Input: part model. Units: mm. Frame: model coordinates. A direction names the side the tool comes from. Coordinates: 2 decimals unless noted, no trailing zeros. Order: outer loops, then holes, each group sorted by start corner. A loop starts at its lowest first (then second) coordinate and runs counter-clockwise, first axis right, second up. Notation, with made-up numbers: (-32.75, 9.25) -> (3.25, 9.25) arc R17 cw to (3.25, 32.25) -> close; hole circle Ø2 at (-38, 47.5). An arc over 180 degrees is marked (long way). Use one line per item in the form item = value. Start each with the question number.
1) Section query B-B on x = 13. Output: boundary loops of the cut face in (y, z), then the cut area to 3 significant figures.
2) Draft query along X for faces 1 (the cylindrical face through (14.9, 27.15, -3.01)), 2 (the flat face through (0, 15, -12)), 3 (the flat face through (22, 15.2, -8.4)), 4 (the cylindrical face through (4.168, 14.79, -11.755)). Return one class per face: pulls with the +X half, pulls with the -X half, needs draft (parallel to the pull), parting line crosses it, or undercut.
3) Ray query, line 1 along Z through (x, y) = (18.75, 15); line 2 along X through (y, z) = (23.25, -12.75); line 3 along X through (y, z) = (8.5, -6.25). Return the intervals inside material, ascending.
4) Section query A-A on y = 15. Output: boundary loops of the cut face in (x, z), then the cut area to 3 significant figures.
5) Access query for faces 5 (the flat face through (15, 15, -13.5)), 6 (the flat face through (8, 15.2, -8.4)), 7 (the flat face through (26, 15, -10)). Directions: +Z, -Z, +X, -X, +Y, -Y. A direction counts if a zero-diameter tool reaches every point of the face in a straight line with its end or side. Return the directions, or none.
6) Section query D-D on y = 22.5. Output: boundary loops of the cut face in (x, z), then the cut area to 3 significant figures.
7) Section query C-C on z = -5. Output: boundary loops of the cut face in (x, y).
8) Pin query (flat end, axial travel): pin 1 (3 mm diameter, centred on x = 9.5, y = 13, fed in from -Z); pin 2 (2 mm diameter, centred on x = 26.5, y = 24, fed in from -Z); pin 3 (8 mm diameter, centred on y = 20.5, z = -4.5, fed in from -X). Return the tip coordinate at first contact, or that it passes through.
from build123d import *

# Parameters (mm, degrees)
BOSS_EXTRUDE1_DEPTH     = 30
CUT_EXTRUDE2_DEPTH      = 46
CUT_EXTRUDE2_DEPTH_BACK = 46
SKETCH3_R               = 3
CUT_EXTRUDE3_DEPTH      = 46
CUT_EXTRUDE3_DEPTH_BACK = 46
SKETCH4_W               = 15.866839518
SKETCH4_H               = 1.721603904
FILLET1_R               = 10
CUT_EXTRUDE4_DEPTH      = 46
CUT_EXTRUDE4_DEPTH_BACK = 46
SKETCH5_W               = 8
SKETCH5_H               = 10


with BuildPart() as part:
    # Sketch1 → Boss-Extrude1 (new body)
    with BuildSketch(Plane(origin=(0, 0, 0), x_dir=(1, 0, 0), z_dir=(0, 1, 0))):
        with BuildLine():
            Line((8.35, 15), (21.65, 15))
            ThreePointArc((21.65, 15), (25, 11.65), (28.35, 15))
            Line((28.35, 15), (30, 15))
            Line((30, 15), (30, 0))
            Line((30, 0), (0, 0))
            Line((0, 0), (0, 15))
            Line((0, 15), (1.65, 15))
            ThreePointArc((1.65, 15), (5, 11.65), (8.35, 15))
        make_face()
    extrude(amount=BOSS_EXTRUDE1_DEPTH)

    # Sketch3 → Cut-Extrude2 (cut, two sides: drawn at the far end of the back side and taken through both)
    with BuildSketch(Plane.ZY.offset(-CUT_EXTRUDE2_DEPTH_BACK)):
        with Locations((-5, 15)):
            Circle(SKETCH3_R)
    extrude(amount=CUT_EXTRUDE2_DEPTH + CUT_EXTRUDE2_DEPTH_BACK, mode=Mode.SUBTRACT)

    # Sketch4 → Cut-Extrude3 (cut, two sides: drawn at the far end of the back side and taken through both)
    with BuildSketch(Plane.XZ.offset(-CUT_EXTRUDE3_DEPTH_BACK)):
        with Locations((14.711914925, -14.360801952)):
            Rectangle(SKETCH4_W, SKETCH4_H)
    extrude(amount=CUT_EXTRUDE3_DEPTH + CUT_EXTRUDE3_DEPTH_BACK, mode=Mode.SUBTRACT)

    # Fillet1
    fillet1_edges = [part.edges().sort_by_distance(p)[0] for p in [
        (15, 0, 0),
        (15, 30, 0),
    ]]
    fillet(fillet1_edges, radius=FILLET1_R)

    # Sketch5 → Cut-Extrude4 (cut, two sides: drawn at the far end of the back side and taken through both)
    with BuildSketch(Plane.XZ.offset(-CUT_EXTRUDE4_DEPTH_BACK)):
        with Locations((4, -5)):
            Rectangle(SKETCH5_W, SKETCH5_H)
        with Locations((26, -5)):
            Rectangle(SKETCH5_W, SKETCH5_H)
    extrude(amount=CUT_EXTRUDE4_DEPTH + CUT_EXTRUDE4_DEPTH_BACK, mode=Mode.SUBTRACT)


solid = part.part
Answers below:
q1.outline = (0, -13.5) -> (30, -13.5) -> (30, -10) arc R10 ccw to (20, 0) -> (10, 0) arc R10 ccw to (0, -10) -> close; hole circle Ø6 at (15, -5)
q1.area = 334 mm^2
q2.face_1 = needs draft
q2.face_2 = pulls with the -X half
q2.face_3 = pulls with the +X half
q2.face_4 = undercut
q3.line_1 = -13.5 to -8, -2 to 0
q3.line_2 = 0 to 2.52, 7.48 to 22.52, 27.48 to 30
q3.line_3 = 8 to 22
q4.outline = (0, -15) -> (1.65, -15) arc R3.35 cw to (8, -13.5) -> (22, -13.5) arc R3.35 cw to (28.35, -15) -> (30, -15) -> (30, -10) -> (22, -10) -> (22, -8) -> (8, -8) -> (8, -10) -> (0, -10) -> close; (8, -2) -> (22, -2) -> (22, 0) -> (8, 0) -> close
q4.area = 150 mm^2
q5.face_5 = -Z, +Y, -Y
q5.face_6 = +Z, -X, +Y, -Y
q5.face_7 = +Z, +X, +Y, -Y
q6.outline = (0, -15) -> (1.65, -15) arc R3.35 cw to (8, -13.5) -> (22, -13.5) arc R3.35 cw to (28.35, -15) -> (30, -15) -> (30, -10) -> (22, -10) -> (22, -0.32) -> (8, -0.32) -> (8, -10) -> (0, -10) -> close
q6.area = 230 mm^2
q7.outline = (8, 1.34) -> (22, 1.34) -> (22, 12) -> (8, 12) -> close; (8, 18) -> (22, 18) -> (22, 28.66) -> (8, 28.66) -> close
q8.pin_1 = -13.5
q8.pin_2 = -12.77
q8.pin_3 = 8
